```python
from build123d import *

# Parameters (mm, degrees)
F0_W      = 45
F0_H      = 30
F0_R      = 1
F0_R_2    = 1.5
F1_DEPTH  = 5
F2_R      = 1
F3_T      = 1
F4_W      = 3.2
F4_H      = 8.1
F5_DEPTH  = 25
F6_R      = 1
F7_DEPTH  = 2.2
F10_DEPTH = 5
F11_R     = 0.75
F12_DEPTH = 2.2
F13_W     = 4
F13_H     = 2
F14_DEPTH = 4


# Not quite as in the source:
# - a shell that OpenCascade refuses in one call is made with other operations: the cavity is built on its own and cut out


with BuildPart() as f1:
    # F0 (on Front) → F1 (new body)
    with BuildSketch(Plane.XZ):
        Rectangle(F0_W, F0_H)
        with Locations((9.5, -5.5)):
            Circle(F0_R, mode=Mode.SUBTRACT)
        with Locations((-10, 0)):
            Circle(F0_R, mode=Mode.SUBTRACT)
        with Locations((9.5, 0)):
            Circle(F0_R_2, mode=Mode.SUBTRACT)
        with Locations((-10, 0)):
            Circle(F0_R)
    extrude(amount=F1_DEPTH)

    # F2
    f2_edges = [f1.edges().sort_by_distance(p)[0] for p in [
        (-22.5, -2.5, -15),
        (22.5, -2.5, -15),
        (22.5, -2.5, 15),
        (-22.5, -2.5, 15),
    ]]
    fillet(f2_edges, radius=F2_R)

    # F3: shell of thickness 1, made by hand


with BuildPart() as f3_core1:
    # F3_t2: copy of F1
    add(f1.part)

    # the walls: a layer under each face that stays
    f3_faces = [f3_core1.faces().sort_by_distance(p)[0] for p in [
        (0, -2.5, -15),
        (0, 0, 0),
        (-22.5, -2.5, 0),
        (22.5, -2.5, 0),
        (0, -2.5, 15),
    ]]
    thicken(f3_faces, amount=-F3_T, mode=Mode.SUBTRACT)


with BuildPart() as f1_1:
    add(f1.part)

    # what is left inside the walls is the cavity
    f3_cavity = [f3_core1.part.solids().sort_by_distance(p)[0] for p in [
        (0, -1.01, -4.666667),
    ]]
    add(f3_cavity, mode=Mode.SUBTRACT)

    # F4 (on face) → F5 (cut)
    with BuildSketch(Plane.YZ.offset(-21.5)):
        with Locations((-2.6, 0)):
            Rectangle(F4_W, F4_H)
    extrude(amount=-F5_DEPTH, mode=Mode.SUBTRACT)

    # F6 (on face) → F7 (join)
    with BuildSketch(Plane.XZ.offset(1)):
        with Locations((-10, 0)):
            Circle(F6_R)
    extrude(amount=F7_DEPTH)

    # F9 (on Top) → F10 (join, symmetric)
    with BuildSketch(Plane.XY):
        Polygon((16.1, 0), (14.1, 0), (14.1, -5), (13.4, -5), (14.1, -7), (16.1, -7), align=None)
    extrude(amount=F10_DEPTH, both=True)

    # F11 (on face) → F12 (join, through all)
    with BuildSketch(Plane.XZ.offset(1)):
        with Locations((12.5, 0)):
            Circle(F11_R)
    extrude(amount=F12_DEPTH)

    # F13 (on face) → F14 (join, through all)
    with BuildSketch(Plane.XZ.offset(1)):
        with Locations((7.1361453363, 10)):
            Rectangle(F13_W, F13_H)
        with Locations((7.1361453363, -10)):
            Rectangle(F13_W, F13_H)
    extrude(amount=F14_DEPTH)


solid = f1_1.part
```
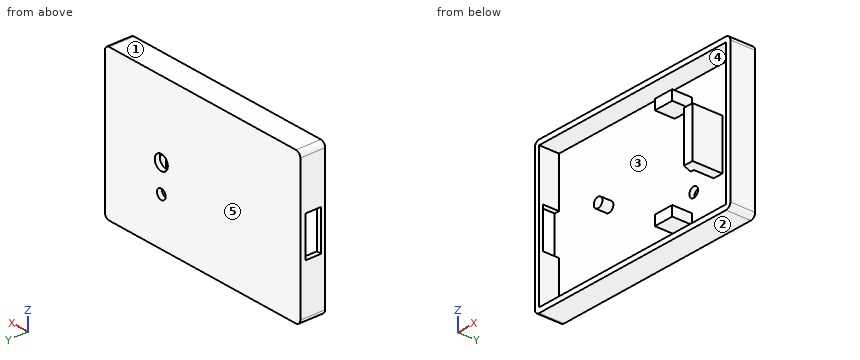
Here's how the part is built. I have some questions about the finished solid (model axes, mm). Face numbers are marked on the shaded views. A direction names the side the tool comes from. Coordinates: 2 decimals unless noted, no trailing zeros. Loops run counter-clockwise (first coordinate to the right, second up) from the corner with the lowest first, then second, coordinate; pieces in that order, holes last. Notation, with made-up numbers: (56.5, 65) - (89.5, 65) arc R25 ccw to (89.5, 77) - close; hole circle Ø7 at (-12, 27.25). An arc over 180 degrees is marked (long way). Answer as CSV lines item,"result".
Q1. If we section it at D-D, the plane z = -5.5: Write out the boundary of the cut face in (x, y).
Response:
outline,"(-22.5, -5) - (-21.5, -5) - (-21.5, -1) - (8.5, -1) - (8.5, 0) - (-22.5, 0) - close; (10.5, -1) - (21.5, -1) - (21.5, -5) - (22.5, -5) - (22.5, 0) - (10.5, 0) - close"
Q2. For pin 1 (2 mm diameter, centred on x = -1.5, z = -7, fed in from -Y), with a flat end and sliding along its axis, tell me the tip position at first contact or that it passes through.
Response:
pin 1,"y = -1"
Q3. For the marked faces 4 and 5, which set-ups out of +Z, -Z, +X, -X, +Y, -Y let a thin tool reach every point of the face, with its end or its side?
Response:
face 4,"-Y"
face 5,"+Z, -Z, +X, -X, +Y"
Q4. If we section it at C-C, the plane x = -1: Write out the boundary of the cut face in (y, z), and give its area (3 significant figures).
Response:
outline,"(-5, -15) - (0, -15) - (0, 15) - (-5, 15) - (-5, 14) - (-1, 14) - (-1, -14) - (-5, -14) - close"
area,"38.0 mm2"
Q5. If I drill on L1, parallel to X at y = -1.25, z = -4.5; L2, parallel to Z at x = 7.5, y = -3.5; L3, parallel to Z at x = 9.5, y = -0.8, over which ranges is the centre line in solid material (lowest first)? Write a range as [from, to].
Response:
L1,"[-22.5, -21.5], [14.1, 16.1], [21.5, 22.5]"
L2,"[-15, -14], [-11, -9], [9, 11], [14, 15]"
L3,"[-15, -6.5], [-4.5, -1.5], [1.5, 15]"
Q6. If we section it at A-A, the plane z = 0: Write out the boundary of the cut face in (x, y), and give its area (3 significant figures).
Response:
outline,"(-22.5, -5) - (-21.5, -5) - (-21.5, -4.2) - (-22.5, -4.2) - close; (-22.5, -1) - (-11, -1) - (-11, -3.2) - (-9, -3.2) - (-9, -1) - (8, -1) - (8, 0) - (-22.5, 0) - close; (11, -1) - (11.75, -1) - (11.75, -3.2) - (13.25, -3.2) - (13.25, -1) - (14.1, -1) - (14.1, -5) - (13.4, -5) - (14.1, -7) - (16.1, -7) - (16.1, -1) - (21.5, -1) - (21.5, -5) - (22.5, -5) - (22.5, 0) - (11, 0) - close"
area,"67.2 mm2"
Q7. If we section it at B-B, the plane y = -2.5: Give the number of separate pieces and of enclosed holes in the cut face, and give its area (3 significant figures).
Response:
separate pieces,"6"
enclosed holes,"0"
area,"178 mm2"
Q8. We'd pull the mould along Z, two halves only. Please class the marked faces 1, 2 and 3: pulls with the +Z half, pulls with the -Z half, needs draft (parallel to the pull), parting line crosses it, or undercut.
Response:
face 1,"pulls with the +Z half"
face 2,"pulls with the -Z half"
face 3,"undercut"
